```python
from build123d import *

# Parameters (mm, degrees)
SKETCH1_W           = 150
SKETCH1_H           = 160
BOSS_EXTRUDE1_DEPTH = 3.2
CUT_EXTRUDE1_REACH  = 5.2
SKETCH2_R           = 7
SKETCH2_R_2         = 2.75
SKETCH3_R           = 2.15
CUT_EXTRUDE2_DEPTH  = 4.2
CIRPATTERN1_COUNT   = 4
SKETCH5_OUTSIDE_W   = 195.868
SKETCH5_OUTSIDE_H   = 205.868
SKETCH5_OUTSIDE_W_2 = 82
SKETCH5_OUTSIDE_H_2 = 100
CUT_EXTRUDE4_DEPTH  = 10


with BuildPart() as part:
    # Sketch1 → Boss-Extrude1 (new body)
    with BuildSketch(Plane.XY):
        Rectangle(SKETCH1_W, SKETCH1_H)
    extrude(amount=BOSS_EXTRUDE1_DEPTH)

    # Sketch2 → Cut-Extrude1 (cut, up to next)
    with BuildSketch(Plane.XY.offset(3.2), mode=Mode.PRIVATE) as cut_extrude1_sk1:
        with Locations((0, -12)):
            Circle(SKETCH2_R)
    cut_extrude1_tool1 = extrude(cut_extrude1_sk1.sketch, amount=-CUT_EXTRUDE1_REACH, mode=Mode.PRIVATE) & part.part
    add(cut_extrude1_tool1.solids().sort_by_distance((0, -12, 3.2))[0], mode=Mode.SUBTRACT)
    # Sketch2 → Cut-Extrude1 (cut, up to next)
    with BuildSketch(Plane.XY.offset(3.2), mode=Mode.PRIVATE) as cut_extrude1_sk2:
        with Locations((-36, -75)):
            Circle(SKETCH2_R_2)
    cut_extrude1_tool2 = extrude(cut_extrude1_sk2.sketch, amount=-CUT_EXTRUDE1_REACH, mode=Mode.PRIVATE) & part.part
    add(cut_extrude1_tool2.solids().sort_by_distance((-36, -75, 3.2))[0], mode=Mode.SUBTRACT)
    # Sketch2 → Cut-Extrude1 (cut, up to next)
    with BuildSketch(Plane.XY.offset(3.2), mode=Mode.PRIVATE) as cut_extrude1_sk3:
        with Locations((36, -75)):
            Circle(SKETCH2_R_2)
    cut_extrude1_tool3 = extrude(cut_extrude1_sk3.sketch, amount=-CUT_EXTRUDE1_REACH, mode=Mode.PRIVATE) & part.part
    add(cut_extrude1_tool3.solids().sort_by_distance((36, -75, 3.2))[0], mode=Mode.SUBTRACT)

    # Sketch3 → Cut-Extrude2 (cut, through all)
    with BuildSketch(Plane.XY.offset(3.2)):
        with Locations((-8.838834765, -3.161165235)):
            Circle(SKETCH3_R)
    cut_extrude2 = extrude(amount=-CUT_EXTRUDE2_DEPTH, mode=Mode.SUBTRACT)

    # CirPattern1: Cut-Extrude2 ×4 about axis
    cirpattern1_axis = Axis((0, -12, 0), (0, 0, 1))
    for i in range(1, CIRPATTERN1_COUNT):
        add(cut_extrude2.rotate(cirpattern1_axis, i * 360 / CIRPATTERN1_COUNT), mode=Mode.SUBTRACT)

    # Sketch5 outside → Cut-Extrude4 (cut)
    with BuildSketch(Plane.XY.offset(3.2)):
        Rectangle(SKETCH5_OUTSIDE_W, SKETCH5_OUTSIDE_H)
        with Locations((0, -30)):
            Rectangle(SKETCH5_OUTSIDE_W_2, SKETCH5_OUTSIDE_H_2, mode=Mode.SUBTRACT)
    extrude(amount=-CUT_EXTRUDE4_DEPTH, mode=Mode.SUBTRACT)


solid = part.part
```
Input: part model. Units: mm. Frame: model coordinates. Round coordinates to 2 decimals unless told otherwise and drop trailing zeros. Loops run counter-clockwise (first coordinate to the right, second up) from the corner with the lowest first, then second, coordinate; pieces in that order, holes last.
1) Pull-direction query (Y, two-part tool) for faces 1 (the flat face through (-1, 20, 2)), 2 (the cylindrical face through (-1.517, -18.834, 1.622)), 3 (the flat face through (-1, -29, 3.2)), 4 (the flat face through (-1, -80, 2)); classes: released by +Y, released by -Y, zero draft, split by the parting line, or undercut.
Ans:
face 1: released by +Y
face 2: undercut
face 3: zero draft
face 4: released by -Y
2) Section query C-C on y = -75. Return the cut outline in (x, z).
Ans:
outline: (-41, 0) - (-38.75, 0) - (-38.75, 3.2) - (-41, 3.2) - close; (-33.25, 0) - (33.25, 0) - (33.25, 3.2) - (-33.25, 3.2) - close; (38.75, 0) - (41, 0) - (41, 3.2) - (38.75, 3.2) - close
3) Section query D-D on z = 2.4. Return the cut outline in (x, y).
Ans:
outline: (-41, -80) - (41, -80) - (41, 20) - (-41, 20) - close; hole circle Ø5.5 at (-36, -75); hole circle Ø4.3 at (-8.84, -20.84); hole circle Ø4.3 at (-8.84, -3.16); hole circle Ø14 at (0, -12); hole circle Ø4.3 at (8.84, -20.84); hole circle Ø4.3 at (8.84, -3.16); hole circle Ø5.5 at (36, -75)
4) Material intervals for line 1 (X direction, y = -21, z = 0.5); line 2 (Y direction, x = -36, z = 0.8); line 3 (Y direction, x = 7.5, z = 2.95), sorted ascending.
Ans:
line 1: x = -41 to -10.98, -6.69 to 6.69, 10.98 to 41
line 2: y = -80 to -77.75, -72.25 to 20
line 3: y = -80 to -22.52, -19.16 to -4.84, -1.48 to 20
5) Section query B-B on y = -12. Return the cut outline in (x, z).
Ans:
outline: (-41, 0) - (-7, 0) - (-7, 3.2) - (-41, 3.2) - close; (7, 0) - (41, 0) - (41, 3.2) - (7, 3.2) - close
6) Section query A-A on x = 0. Return the cut outline in (y, z).
Ans:
outline: (-80, 0) - (-19, 0) - (-19, 3.2) - (-80, 3.2) - close; (-5, 0) - (20, 0) - (20, 3.2) - (-5, 3.2) - close
7) Pin query (flat end, axial travel): pin 1 (5 mm diameter, centred on x = -8.84, y = -3.16, fed in from +Z). Return the tip coordinate at first contact, or that it passes through.
Ans:
pin 1: stops at z = 3.2
